Verification items for the finished model (mm, model axes). A direction names the side the tool comes from. Round coordinates to 2 decimals unless told otherwise and drop trailing zeros. Write each loop counter-clockwise with the first axis right and the second up, starting at its lowest first coordinate (ties: lowest second). Pieces come first, ordered by that corner, then holes. Notation, with made-up numbers: M -34,-32 L 18,-32 A17 ccw 18,-15 Z; hole C -28.75,48 d8. An arc over 180 degrees is marked long. One line per question, with ' | ' between items. Start each with the question number.
Q1. Gauge pin test, flat ends, axial feed: pin 1 (9 mm diameter, centred on x = 184.15, z = -190.5, fed in from +Y); pin 2 (11 mm diameter, centred on x = 69.5, z = -12.5, fed in from +Y); pin 3 (4 mm diameter, centred on y = 15, z = -76.5, fed in from -X); pin 4 (1.9 mm diameter, centred on x = 131.5, y = 16.5, fed in from +Z). Record the tip position at first contact, or that the pin passes through.
Q2. Thickness scan on line 1 along X through (y, z) = (1.35, -190.5); line 2 along Z through (x, y) = (12.7, 7); line 3 along X through (y, z) = (9, -57.15). Record the ranges inside material, lowest first. Write a range as from..to.
Q3. Cross-section at A-A (x = 211). Record the boundary of the cut face in (y, z), then the cut area to 3 significant figures.
Q4. Tool access check on faces 1 (the face through (25.4, 6, -101)), 2 (the face through (14.9, 4.7, -10.5)), 3 (the face through (0, 7, -135)). Record the directions out of +Z, -Z, +X, -X, +Y, -Y that give a thin tool (end or side, any length) a straight path to the whole face; none if there is none.
Q5. Release check for a two-part mould opening along Z. For faces 4 (the face through (72, 4.7, -10.5)), 5 (the face through (254, 7, -135)) record: released by +Z, released by -Z, zero draft, split by the parting line, or undercut.
Q6. Cross-section at B-B (z = -120). Record the boundary of the cut face in (x, y), then the cut area to 3 significant figures.
from build123d import *

# Parameters (mm, degrees)
SKETCH1_W                      = 254
SKETCH1_H                      = 203.2
SKETCH1_R                      = 3.05
SKETCH1_W_2                    = 203.2
SKETCH1_H_2                    = 152.4
BOSS_EXTRUDE1_DEPTH            = 12.7
SKETCH5_W                      = 254
SKETCH5_H                      = 19.05
BOSS_EXTRUDE3_DEPTH            = 12.7
SKETCH6_R                      = 2
CUT_EXTRUDE2_DEPTH             = 4.5
SKETCH7_R                      = 1.75
CUT_EXTRUDE3_DEPTH             = 4.5
SKETCH8_R                      = 1.75
SKETCH8_W                      = 14.64249385
SKETCH8_H                      = 9.353844035
SKETCH8_W_2                    = 16.268144154
SKETCH8_W_3                    = 13.224120591
SKETCH8_H_2                    = 10.411082314
BOSS_EXTRUDE4_DEPTH            = 12.7
SKETCH9_W                      = 254
SKETCH9_H                      = 43.18
SKETCH9_R                      = 1.75
SKETCH9_R_2                    = 1.707438486
BOSS_EXTRUDE5_DEPTH            = 6.35
CBORE_FOR_M5_SHCS2_D           = 5.8
CBORE_FOR_M5_SHCS2_CBORE_D     = 10
CBORE_FOR_M5_SHCS2_CBORE_DEPTH = 8
SKETCH12_R                     = 2
CUT_EXTRUDE4_DEPTH             = 11


with BuildPart() as part:
    # Sketch1 → Boss-Extrude1 (new body)
    with BuildSketch(Plane(origin=(0, 0, 0), x_dir=(1, 0, 0), z_dir=(0, 1, 0))):
        with Locations((127, 101.6)):
            Rectangle(SKETCH1_W, SKETCH1_H)
        with Locations((12.7, 190.5)):
            Circle(SKETCH1_R, mode=Mode.SUBTRACT)
        with Locations((241.3, 190.5)):
            Circle(SKETCH1_R, mode=Mode.SUBTRACT)
        with Locations((241.3, 12.7)):
            Circle(SKETCH1_R, mode=Mode.SUBTRACT)
        with Locations((12.7, 12.7)):
            Circle(SKETCH1_R, mode=Mode.SUBTRACT)
        with Locations((127, 101.6)):
            Rectangle(SKETCH1_W_2, SKETCH1_H_2, mode=Mode.SUBTRACT)
    extrude(amount=BOSS_EXTRUDE1_DEPTH)

    # Sketch5 → Boss-Extrude3 (add)
    with BuildSketch(Plane.XZ):
        with Locations((127, -212.725)):
            Rectangle(SKETCH5_W, SKETCH5_H)
    extrude(amount=-BOSS_EXTRUDE3_DEPTH)

    # Sketch6 → Cut-Extrude2 (cut)
    with BuildSketch(Plane(origin=(0, 12.7, 0), x_dir=(1, 0, 0), z_dir=(0, 1, 0))):
        with Locations((19.924999942, 216.120415829)):
            Circle(SKETCH6_R)
        with Locations((34.924999942, 216.120415829)):
            Circle(SKETCH6_R)
        with Locations((49.936813619, 216.120415829)):
            Circle(SKETCH6_R)
        with Locations((204.063186381, 216.120415829)):
            Circle(SKETCH6_R)
        with Locations((219.075000058, 216.120415829)):
            Circle(SKETCH6_R)
        with Locations((234.075000058, 216.120415829)):
            Circle(SKETCH6_R)
    extrude(amount=-CUT_EXTRUDE2_DEPTH, mode=Mode.SUBTRACT)

    # Sketch7 → Cut-Extrude3 (cut)
    with BuildSketch(Plane(origin=(0, 8.2, 0), x_dir=(1, 0, 0), z_dir=(0, 1, 0))):
        with Locations((19.924999942, 216.120415829)):
            Circle(SKETCH7_R)
        with Locations((34.924999942, 216.120415829)):
            Circle(SKETCH7_R)
        with Locations((49.936813619, 216.120415829)):
            Circle(SKETCH7_R)
        with Locations((204.063186381, 216.120415829)):
            Circle(SKETCH7_R)
        with Locations((219.075000058, 216.120415829)):
            Circle(SKETCH7_R)
        with Locations((234.075000058, 216.120415829)):
            Circle(SKETCH7_R)
    extrude(amount=-CUT_EXTRUDE3_DEPTH, mode=Mode.SUBTRACT)

    # Sketch8 → Boss-Extrude4 (add)
    with BuildSketch(Plane(origin=(0, 12.7, 0), x_dir=(1, 0, 0), z_dir=(0, 1, 0))):
        Polygon((0, 222.25), (13.150330977, 222.25), (13.150330977, 209.354277193), (243.652075008, 209.354277193), (243.652075008, 222.25), (254, 222.25), (254, 273.05), (0, 273.05), align=None)
        with Locations((49.936813619, 236.120415829)):
            Circle(SKETCH8_R, mode=Mode.SUBTRACT)
        with Locations((34.924999942, 236.120415829)):
            Circle(SKETCH8_R, mode=Mode.SUBTRACT)
        with Locations((19.924999942, 236.120415829)):
            Circle(SKETCH8_R, mode=Mode.SUBTRACT)
        with Locations((204.063186381, 236.120415829)):
            Circle(SKETCH8_R, mode=Mode.SUBTRACT)
        with Locations((219.075000058, 236.120415829)):
            Circle(SKETCH8_R, mode=Mode.SUBTRACT)
        with Locations((234.075000058, 236.120415829)):
            Circle(SKETCH8_R, mode=Mode.SUBTRACT)
        with Locations((12.603753017, 189.643423316)):
            Rectangle(SKETCH8_W, SKETCH8_H)
        with Locations((239.165048572, 189.643423316)):
            Rectangle(SKETCH8_W_2, SKETCH8_H)
        with Locations((240.687060353, 12.36659945)):
            Rectangle(SKETCH8_W_3, SKETCH8_H_2)
        with Locations((12.603753017, 12.36659945)):
            Rectangle(SKETCH8_W, SKETCH8_H_2)
    extrude(amount=-BOSS_EXTRUDE4_DEPTH)

    # Sketch9 → Boss-Extrude5 (add)
    with BuildSketch(Plane(origin=(0, 12.7, 0), x_dir=(1, 0, 0), z_dir=(0, 1, 0))):
        with Locations((127, 251.46)):
            Rectangle(SKETCH9_W, SKETCH9_H)
        with Locations((19.924999942, 236.120415829)):
            Circle(SKETCH9_R, mode=Mode.SUBTRACT)
        with Locations((34.924999942, 236.120415829)):
            Circle(SKETCH9_R_2, mode=Mode.SUBTRACT)
        with Locations((49.936813619, 236.120415829)):
            Circle(SKETCH9_R, mode=Mode.SUBTRACT)
        with Locations((204.063186381, 236.120415829)):
            Circle(SKETCH9_R, mode=Mode.SUBTRACT)
        with Locations((219.075000058, 236.120415829)):
            Circle(SKETCH9_R, mode=Mode.SUBTRACT)
        with Locations((234.075000058, 236.120415829)):
            Circle(SKETCH9_R, mode=Mode.SUBTRACT)
    extrude(amount=BOSS_EXTRUDE5_DEPTH)

    # CBORE for M5 SHCS2 (through all)
    with Locations(Plane(origin=(0, 12.7, 0), x_dir=(1, 0, 0), z_dir=(0, 1, 0))):
        with Locations((12.7, 101.6), (241.3, 190.5), (12.7, 12.7), (12.7, 190.5), (127, 190.5), (127, 12.7), (241.3, 12.7), (184.15, 190.5), (184.15, 12.7), (69.85, 12.7), (69.85, 190.5), (12.7, 146.05), (12.7, 57.15), (241.3, 57.15), (241.3, 146.05), (241.3, 101.6)):
            CounterBoreHole(CBORE_FOR_M5_SHCS2_D / 2, CBORE_FOR_M5_SHCS2_CBORE_D / 2, CBORE_FOR_M5_SHCS2_CBORE_DEPTH)

    # Sketch12 → Cut-Extrude4 (cut)
    with BuildSketch(Plane.XZ):
        with Locations((219.075000058, -236.120415829)):
            Circle(SKETCH12_R)
        with Locations((204.063186381, -236.120415829)):
            Circle(SKETCH12_R)
        with Locations((49.936813619, -236.120415829)):
            Circle(SKETCH12_R)
        with Locations((34.924999942, -236.120415829)):
            Circle(SKETCH12_R)
        with Locations((19.924999942, -236.120415829)):
            Circle(SKETCH12_R)
        with Locations((234.075000058, -236.120415829)):
            Circle(SKETCH12_R)
    extrude(amount=-CUT_EXTRUDE4_DEPTH, mode=Mode.SUBTRACT)


solid = part.part
Determined:
1) pin 1: stops at y = 4.7 | pin 2: stops at y = 12.7 | pin 3: passes through | pin 4: stops at z = -229.87
2) line 1: x = 0..9.8, 15.6..66.95, 72.75..124.1, 129.9..181.25, 187.05..238.4, 244.2..254 | line 2: z = -273.05..-195.5, -185.5..-151.05, -141.05..-106.6, -96.6..-62.15, -52.15..-17.7, -7.7..0 | line 3: x = 0..7.7, 17.7..25.4, 228.6..236.3, 246.3..254
3) outline: M 0,-273.05 L 19.05,-273.05 L 19.05,-229.87 L 12.7,-229.87 L 12.7,-177.8 L 0,-177.8 Z; M 0,-25.4 L 12.7,-25.4 L 12.7,0 L 0,0 Z | area: 1,810 mm²
4) face 1: +Y, -Y | face 2: +Y | face 3: +Z, -Z, -X, +Y, -Y
5) face 4: undercut | face 5: zero draft
6) outline: M 0,0 L 25.4,0 L 25.4,12.7 L 0,12.7 Z; M 228.6,0 L 254,0 L 254,12.7 L 228.6,12.7 Z | area: 645 mm²
